Source: CAD feature listing. Evaluate the final solid. Frame: model axes, mm. Face numbers are marked on the shaded views. A direction names the side the tool comes from. Give positions to 0.01 mm unless a question says otherwise; leave off trailing zeros. Loops run counter-clockwise (first coordinate to the right, second up) from the corner with the lowest first, then second, coordinate; pieces in that order, holes last.
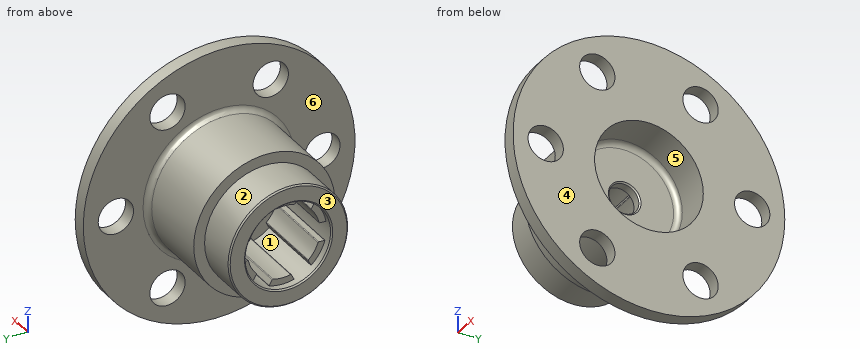
```python
from build123d import *

# Parameters (mm, degrees)
SZKIC4_R                    = 6.5
WYTNIJ_WYCI_GNI_CIE1_DEPTH  = 10
SZYK_KO_OWY1_COUNT          = 6
ZAOKR_GLENIE1_R             = 2
SZKIC6_R                    = 16.5
DODANIE_WYCI_GNI_CIE1_DEPTH = 26
SFAZOWANIE1_SIZE            = 0.5


with BuildPart() as part:
    # Szkic2 → Obrót1 (revolve)
    with BuildSketch(Plane.XY):
        Polygon((0, 15.75), (29, 15.75), (29, 5.5), (33, 5.5), (33, 20), (48, 20), (48, 50), (43, 50), (43, 26), (15, 26), (15, 22), (0, 22), align=None)
    revolve(axis=Axis((0, 0, 0), (1, 0, 0)))

    # Szkic4 → Wytnij-wyciągnięcie1 (cut)
    with BuildSketch(Plane(origin=(48, 0, 0), x_dir=(0, 0, -1), z_dir=(1, 0, 0))):
        with Locations((0, 38)):
            Circle(SZKIC4_R)
    wytnij_wyci_gni_cie1 = extrude(amount=-WYTNIJ_WYCI_GNI_CIE1_DEPTH, mode=Mode.SUBTRACT)

    # Szyk kołowy1: Wytnij-wyciągnięcie1 ×6 about axis
    szyk_ko_owy1_axis = Axis((0, 0, 0), (1, 0, 0))
    for i in range(1, SZYK_KO_OWY1_COUNT):
        add(wytnij_wyci_gni_cie1.rotate(szyk_ko_owy1_axis, i * 360 / SZYK_KO_OWY1_COUNT), mode=Mode.SUBTRACT)

    # Zaokrąglenie1
    zaokr_glenie1_edges = [part.edges().sort_by_distance(p)[0] for p in [
        (33, -20, 0),
        (43, -26, 0),
    ]]
    fillet(zaokr_glenie1_edges, radius=ZAOKR_GLENIE1_R)

    # Szkic6 → Dodanie-wyciągnięcie1 (add)
    with BuildSketch(Plane.ZY.offset(-29)):
        Circle(SZKIC6_R)
        with BuildLine():
            Line((-4.32821665, -14.980955932), (-4.33920313, -15.180955932))
            ThreePointArc((-4.33920313, -15.180955932), (-4.301860669, -15.308717905), (-4.192604113, -15.384748071))
            ThreePointArc((-4.192604113, -15.384748071), (-0.874869369, -15.926290292), (2.482220063, -15.751412191))
            ThreePointArc((2.482220063, -15.751412191), (2.599147134, -15.687806835), (2.650259222, -15.564903882))
            Line((2.650259222, -15.564903882), (2.661245702, -15.364903882))
            Line((2.661245702, -15.364903882), (2.775629759, -13.282634507))
            ThreePointArc((2.775629759, -13.282634507), (2.845574347, -13.106003698), (3.007591812, -13.006801739))
            ThreePointArc((3.007591812, -13.006801739), (6.030810048, -11.910156597), (8.704052682, -10.122349871))
            ThreePointArc((8.704052682, -10.122349871), (8.879904359, -10.050468889), (9.063673937, -10.098629351))
            Line((9.063673937, -10.098629351), (10.809780085, -11.238823538))
            Line((10.809780085, -11.238823538), (10.977491925, -11.348338109))
            ThreePointArc((10.977491925, -11.348338109), (11.106808271, -11.379879576), (11.227280604, -11.323275705))
            ThreePointArc((11.227280604, -11.323275705), (13.355137297, -8.720804245), (14.882233134, -5.726040463))
            ThreePointArc((14.882233134, -5.726040463), (14.885612816, -5.592975971), (14.80473178, -5.487260129))
            Line((14.80473178, -5.487260129), (14.63701994, -5.377745558))
            Line((14.63701994, -5.377745558), (12.890913792, -4.237551371))
            ThreePointArc((12.890913792, -4.237551371), (12.772919318, -4.088662177), (12.768016635, -3.898749956))
            ThreePointArc((12.768016635, -3.898749956), (13.3299032, -0.732243591), (13.118238475, 2.476755803))
            ThreePointArc((13.118238475, 2.476755803), (13.143913557, 2.664988314), (13.27750653, 2.800057205))
            Line((13.27750653, 2.800057205), (15.137996735, 3.742132394))
            Line((15.137996735, 3.742132394), (15.316695056, 3.832617823))
            ThreePointArc((15.316695056, 3.832617823), (15.40866894, 3.928838329), (15.419884717, 4.061472366))
            ThreePointArc((15.419884717, 4.061472366), (14.230006666, 7.205486047), (12.400013071, 10.025371728))
            ThreePointArc((12.400013071, 10.025371728), (12.286465682, 10.094830864), (12.154472559, 10.077643754))
            Line((12.154472559, 10.077643754), (11.975774238, 9.987158325))
            Line((11.975774238, 9.987158325), (10.115284033, 9.045083136))
            ThreePointArc((10.115284033, 9.045083136), (9.927344971, 9.017341522), (9.760424822, 9.108051784))
            ThreePointArc((9.760424822, 9.108051784), (7.299093152, 11.177913005), (4.414185793, 12.599105674))
            ThreePointArc((4.414185793, 12.599105674), (4.264009198, 12.715457202), (4.213832593, 12.898686556))
            Line((4.213832593, 12.898686556), (4.32821665, 14.980955932))
            Line((4.32821665, 14.980955932), (4.33920313, 15.180955932))
            ThreePointArc((4.33920313, 15.180955932), (4.301860669, 15.308717905), (4.192604113, 15.384748071))
            ThreePointArc((4.192604113, 15.384748071), (0.874869369, 15.926290292), (-2.482220063, 15.751412191))
            ThreePointArc((-2.482220063, 15.751412191), (-2.599147134, 15.687806835), (-2.650259222, 15.564903882))
            Line((-2.650259222, 15.564903882), (-2.661245702, 15.364903882))
            Line((-2.661245702, 15.364903882), (-2.775629759, 13.282634507))
            ThreePointArc((-2.775629759, 13.282634507), (-2.845574347, 13.106003698), (-3.007591812, 13.006801739))
            ThreePointArc((-3.007591812, 13.006801739), (-6.030810048, 11.910156597), (-8.704052682, 10.122349871))
            ThreePointArc((-8.704052682, 10.122349871), (-8.879904359, 10.050468889), (-9.063673937, 10.098629351))
            Line((-9.063673937, 10.098629351), (-10.809780085, 11.238823538))
            Line((-10.809780085, 11.238823538), (-10.977491925, 11.348338109))
            ThreePointArc((-10.977491925, 11.348338109), (-11.106808271, 11.379879576), (-11.227280604, 11.323275705))
            ThreePointArc((-11.227280604, 11.323275705), (-13.355137297, 8.720804245), (-14.882233134, 5.726040463))
            ThreePointArc((-14.882233134, 5.726040463), (-14.885612816, 5.592975971), (-14.80473178, 5.487260129))
            Line((-14.80473178, 5.487260129), (-14.63701994, 5.377745558))
            Line((-14.63701994, 5.377745558), (-12.890913792, 4.237551371))
            ThreePointArc((-12.890913792, 4.237551371), (-12.772919318, 4.088662177), (-12.768016635, 3.898749956))
            ThreePointArc((-12.768016635, 3.898749956), (-13.3299032, 0.732243591), (-13.118238475, -2.476755803))
            ThreePointArc((-13.118238475, -2.476755803), (-13.143913557, -2.664988314), (-13.27750653, -2.800057205))
            Line((-13.27750653, -2.800057205), (-15.137996735, -3.742132394))
            Line((-15.137996735, -3.742132394), (-15.316695056, -3.832617823))
            ThreePointArc((-15.316695056, -3.832617823), (-15.40866894, -3.928838329), (-15.419884717, -4.061472366))
            ThreePointArc((-15.419884717, -4.061472366), (-14.230006666, -7.205486047), (-12.400013071, -10.025371728))
            ThreePointArc((-12.400013071, -10.025371728), (-12.286465682, -10.094830864), (-12.154472559, -10.077643754))
            Line((-12.154472559, -10.077643754), (-11.975774238, -9.987158325))
            Line((-11.975774238, -9.987158325), (-10.115284033, -9.045083136))
            ThreePointArc((-10.115284033, -9.045083136), (-9.927344971, -9.017341522), (-9.760424822, -9.108051784))
            ThreePointArc((-9.760424822, -9.108051784), (-7.299093152, -11.177913005), (-4.414185793, -12.599105674))
            ThreePointArc((-4.414185793, -12.599105674), (-4.264009198, -12.715457202), (-4.213832593, -12.898686556))
            Line((-4.213832593, -12.898686556), (-4.32821665, -14.980955932))
        make_face(mode=Mode.SUBTRACT)
    extrude(amount=DODANIE_WYCI_GNI_CIE1_DEPTH)

    # Sfazowanie1
    sfazowanie1_edges = [part.edges().sort_by_distance(p)[0] for p in [
        (33, -5.5, 0),
        (29, -5.5, 0),
        (0, -15.75, 0),
        (0, -22, 0),
    ]]
    chamfer(sfazowanie1_edges, length=SFAZOWANIE1_SIZE)


solid = part.part
```
(1) Reachability of the marked faces 4, 5 and 6 from +Z, -Z, +X, -X, +Y, -Y: full face, straight path, thin tool, end or side. Return the list, or none.
A:
face 4: +Z, -Z, +X, +Y, -Y
face 5: +X
face 6: -X
(2) Section C-C, the plane x = 44.5. Return the cut outline in (y, z), then the cut area to 3 significant figures.
A:
outline: circle Ø100 at (0, 0); hole circle Ø13 at (-38, 0); hole circle Ø13 at (-19, -32.91); hole circle Ø13 at (-19, 32.91); hole circle Ø40 at (0, 0); hole circle Ø13 at (19, -32.91); hole circle Ø13 at (19, 32.91); hole circle Ø13 at (38, 0)
area: 5,800 mm2
(3) First-contact query: pin 1 (17 mm diameter, centred on y = 19, z = -32.91, fed in from +X); pin 2 (2.5 mm diameter, centred on y = 12.5, z = -5, fed in from -X); pin 3 (10.5 mm diameter, centred on y = -19, z = 32.91, fed in from +X); pin 4 (1.8 mm diameter, centred on y = -13, z = -7.5, fed in from -X). Flat tips, straight axial feed; report the tip coordinate or a pass-through.
A:
pin 1: stops at x = 48
pin 2: stops at x = 3
pin 3: passes through
pin 4: stops at x = 0.34
(4) Section A-A, the plane y = 38. Return the cut outline in (x, z), then the cut area to 3 significant figures.
A:
outline: (43, -32.5) - (48, -32.5) - (48, -6.5) - (43, -6.5) - close; (43, 6.5) - (48, 6.5) - (48, 32.5) - (43, 32.5) - close
area: 260 mm2
(5) Section B-B, the plane z = 0. Count the separate pieces of the cut face and the enclosed holes in it, then the cut area to 3 significant figures.
A:
separate pieces: 4
enclosed holes: 0
area: 931 mm2
(6) Mould query, pull axis Z, two halves, no side actions, for the marked faces 1, 2 and 3. Classes: pulls with the +Z half, pulls with the -Z half, needs draft (parallel to the pull), parting line crosses it, or undercut.
A:
face 1: undercut
face 2: parting line crosses it
face 3: needs draft
(7) Section D-D, the plane z = -34. Return the cut outline in (x, y), then the cut area to 3 significant figures.
A:
outline: (43, -36.66) - (48, -36.66) - (48, -25.41) - (43, -25.41) - close; (43, -12.59) - (48, -12.59) - (48, 12.59) - (43, 12.59) - close; (43, 25.41) - (48, 25.41) - (48, 36.66) - (43, 36.66) - close
area: 238 mm2
(8) Ray query, line 1 along Z through (x, y) = (20.5, 7.5); line 2 along X through (y, z) = (13.5, 18.5); line 3 along Y through (x, z) = (7, 5.5). Return the intervals inside material, ascending.
A:
line 1: z = -24.89 to -13.85, 13.85 to 24.89
line 2: x = 15 to 48
line 3: y = -21.3 to -12.16, 12.16 to 21.3
